Can you work these out from the model? Positions are in its coordinate system, mm. A direction names the side the tool comes from. Coordinates: 2 decimals unless noted, no trailing zeros. Write each loop counter-clockwise with the first axis right and the second up, starting at its lowest first coordinate (ties: lowest second). Pieces come first, ordered by that corner, then holes. Notation, with made-up numbers: M 80.5,17 L 99.5,17 A13 cw 99.5,31 Z; hole C 48.25,76.25 d9. An arc over 180 degrees is marked long. Answer as a JSON object with one key per item and string values. Group by question number.
from build123d import *

# Parameters (mm, degrees)
SKETCH2_W               = 15
SKETCH2_H               = 3
BOSS_EXTRUDE1_DEPTH     = 5
SKETCH4_W               = 6
SKETCH4_H               = 7.676307803
CUT_EXTRUDE1_DEPTH      = 10
FILLET2_R               = 10
FILLET3_R               = 10
CUT_EXTRUDE2_DEPTH      = 80.142875261
CUT_EXTRUDE2_DEPTH_BACK = 80.142875261
BOSS_EXTRUDE2_DEPTH     = 4


with BuildPart() as part:
    # Sketch2 → Revolve1 (revolve)
    with BuildSketch(Plane.XY, mode=Mode.PRIVATE) as revolve1_sk:
        with BuildLine():
            ThreePointArc((-10, 14.97), (-9.414213562, 16.384213562), (-8, 16.97))
            Line((-8, 16.97), (0, 16.97))
            Line((0, 16.97), (0, 14.97))
            Line((0, 14.97), (0, 13.97))
            Line((0, 13.97), (0, 5))
            Line((0, 5), (0, 3))
            Line((0, 3), (-15, 3))
            Line((-15, 3), (-13, 5))
            ThreePointArc((-13, 5), (-13.688325627, 10.216881481), (-10, 13.97))
            Line((-10, 13.97), (-10, 14.97))
        make_face()
        with Locations((-7.5, 1.5)):
            Rectangle(SKETCH2_W, SKETCH2_H)
    revolve(revolve1_sk.sketch.rotate(Axis((0, 5, 0), (0, 1, 0)), 270), axis=Axis((0, 5, 0), (0, 1, 0)))

    # Sketch3 → Boss-Extrude1 (add, symmetric)
    with BuildSketch(Plane.XY):
        with BuildLine():
            ThreePointArc((0, 44.765662821), (8.195556272, 39.305823104), (10.13, 29.65))
            ThreePointArc((10.13, 29.65), (9.728307106, 26.745012699), (8.67, 24.01))
            ThreePointArc((8.67, 24.01), (7.233209761, 20.609032371), (6.61, 16.97))
            Line((6.61, 16.97), (-6.61, 16.97))
            ThreePointArc((-6.61, 16.97), (-7.233209761, 20.609032371), (-8.67, 24.01))
            ThreePointArc((-8.67, 24.01), (-13.717238878, 50.759844741), (-1.33, 75))
            Line((-1.33, 75), (0, 67.29))
            Line((0, 67.29), (8.67, 64.56))
            Line((8.67, 64.56), (8.14100346, 62.88))
            Line((8.14100346, 62.88), (20.337027919, 55.57))
            Line((20.337027919, 55.57), (20.337027919, 53.136090211))
            Line((20.337027919, 53.136090211), (17.983362656, 53.773319693))
            Line((17.983362656, 53.773319693), (20.337027919, 52.381882691))
            Line((20.337027919, 52.381882691), (20.337027919, 50.702180422))
            Line((20.337027919, 50.702180422), (1.260409295, 53.136090211))
            Line((1.260409295, 53.136090211), (-1.816215968, 50.059464948))
            Line((-1.816215968, 50.059464948), (0, 44.765662821))
        make_face()
    extrude(amount=BOSS_EXTRUDE1_DEPTH, both=True)

    # Sketch4 → Cut-Extrude1 (cut)
    with BuildSketch(Plane(origin=(0, 0, 0), x_dir=(0, 0, -1), z_dir=(1, 0, 0))):
        with Locations((0, 72.886493521)):
            Rectangle(SKETCH4_W, SKETCH4_H)
    extrude(amount=-CUT_EXTRUDE1_DEPTH, mode=Mode.SUBTRACT)

    # Fillet2
    # the kernel refuses this fillet: 10 mm, written as the material it takes off along each edge
    with BuildSketch(Plane(origin=(20.337027919, 55.57, 17.159563067), x_dir=(-0.8577290982340794, 0.5141019296234484, 0), z_dir=(0, 0, -1))) as fillet2_piece_1:
        with BuildLine():
            CenterArc((4.863825227, -10), FILLET2_R, 90, 37.698787392)
            Line((-1.251277719, -2.087635248), (-1.373579778, -1.929387953))
            ThreePointArc((-1.373579778, -1.929387953), (-0.797184679, -0.940997238), (-0.17154582, 0.102820386))
            Line((-0.17154582, 0.102820386), (0, 0.2))
            Line((0, 0.2), (4.863825227, 0.2))
            Line((4.863825227, 0.2), (4.863825227, 0))
        make_face()
    extrude(amount=34.319126134, mode=Mode.SUBTRACT)

    # Fillet3
    # the kernel refuses this fillet: 10 mm, written as the material it takes off along each edge
    with BuildSketch(Plane(origin=(20.337027919, 50.702180422, 19.348952899), x_dir=(-0.9919589424380495, 0.12656009053878878, 0), z_dir=(0, 0, -1))) as fillet3_piece_1:
        with BuildLine():
            CenterArc((5.73958116, 10), FILLET3_R, 236.447572357, 33.552427643)
            Line((0.212583271, 1.666195686), (0.102043313, 1.4995196))
            ThreePointArc((0.102043313, 1.4995196), (-0.092100153, 0.858409861), (-0.198391788, 0.025312018))
            Line((-0.198391788, 0.025312018), (0, -0.2))
            Line((0, -0.2), (5.73958116, -0.2))
            Line((5.73958116, -0.2), (5.73958116, 0))
        make_face()
    extrude(amount=38.697905798, mode=Mode.SUBTRACT)

    # Sketch5 → Cut-Extrude2 (cut, two sides: drawn at the far end of the back side and taken through both)
    with BuildSketch(Plane.XY.offset(-CUT_EXTRUDE2_DEPTH_BACK)):
        with BuildLine():
            ThreePointArc((3.123689943, 61.436717182), (5.265012371, 59.692471778), (7.983104726, 59.202953935))
            ThreePointArc((7.983104726, 59.202953935), (6.01602485, 61.326253313), (3.123689943, 61.436717182))
        make_face()
    extrude(amount=CUT_EXTRUDE2_DEPTH + CUT_EXTRUDE2_DEPTH_BACK, mode=Mode.SUBTRACT)

    # Sketch5<3> → Boss-Extrude2 (add, symmetric)
    with BuildSketch(Plane.XY):
        with BuildLine():
            ThreePointArc((3.123689943, 61.436717182), (5.265012371, 59.692471778), (7.983104726, 59.202953935))
            ThreePointArc((7.983104726, 59.202953935), (6.01602485, 61.326253313), (3.123689943, 61.436717182))
        make_face()
    extrude(amount=BOSS_EXTRUDE2_DEPTH, both=True)


solid = part.part
Q1. Will these pins go through, and if not, where does the flat tip stop? pin 1 (0.7 mm diameter, centred on x = 4.5, y = 61, fed in from +Z); pin 2 (3 mm diameter, centred on x = -2.5, y = 73, fed in from +Z); pin 3 (10 mm diameter, centred on x = 13, y = 39.5, fed in from -Z).
Q2. If we section it at B-B on y = 6: List the corners of the cut face in (x, z) for me, and give its area (3 significant figures).
Q3. Please list where these lines run through material, in increasing order: L1, parallel to Y at x = 4, z = -5.25; L2, parallel to Z at x = 1, y = 42; L3, parallel to Y at x = 9, z = -10.25.
Q4. We'd pull the mould along X, two halves only. Please class faces 5 (the cylindrical face through (-7.22, 20.56, 0.07)), 6 (the flat face through (12.097, 60.509, 0.07)), 7 (the cylindrical face through (6.05, 61.31, 4.49)): pulls with the +X half, pulls with the -X half, needs draft (parallel to the pull), parting line crosses it, or undercut.
Q5. On a 3-axis mill with a long thin cutter (end or side, diameter ignored), from which of +Z, -Z, +X, -X, +Y, -Y can I reach the whole of each face in a straight line? I mean faces 1 (the flat face through (-0.256, 51.619, 0.07)), 2 (the flat face through (0, 16.97, 6)), 3 (the flat face through (8.4, 63.7, 0.1)), 4 (the flat face through (6, 60, -4)). Say none if no direction works.
Reply:
{
 "1": {"pin 1": "z = 4", "pin 2": "z = 5", "pin 3": "z = -5"},
 "2": {"outline": "C 0,0 d27.07", "area": "575 mm^2"},
 "3": {"L1": "0 to 16.97", "L2": "-5 to 5", "L3": "0 to 4.36, 6.27 to 10.35"},
 "4": {"face 5": "pulls with the -X half", "face 6": "pulls with the +X half", "face 7": "undercut"},
 "5": {"face 1": "+Z, -Z", "face 2": "+Z, +X, -X, +Y", "face 3": "+Z, -Z, +X", "face 4": "-Z"}
}
